Geometry: final body of the model. Coordinates: model frame, mm. Face numbers are marked on the shaded views. A direction names the side the tool comes from. Round coordinates to 2 decimals unless told otherwise and drop trailing zeros. Order: outer loops, then holes, each group sorted by start corner. A loop starts at its lowest first (then second) coordinate and runs counter-clockwise, first axis right, second up. Notation, with made-up numbers: (73.5, -16) -> (128.5, -16) arc R27 cw to (128.5, 8) -> close; hole circle Ø10 at (-34, -5). An arc over 180 degrees is marked (long way). Put each result on its own line as item: value.
```python
from build123d import *

# Parameters (mm, degrees)
SKETCH1_W           = 4
SKETCH1_H           = 76
SKETCH1_H_2         = 4
SKETCH1_W_2         = 76
BOSS_EXTRUDE1_DEPTH = 150


with BuildPart() as part:
    # Sketch1 → Boss-Extrude1 (new body)
    with BuildSketch(Plane.XY):
        with Locations((0, 2)):
            Rectangle(SKETCH1_W, SKETCH1_H)
        with Locations((0, -38)):
            Rectangle(SKETCH1_W, SKETCH1_H_2)
        with Locations((40, -38)):
            Rectangle(SKETCH1_W_2, SKETCH1_H_2)
    extrude(amount=BOSS_EXTRUDE1_DEPTH)


solid = part.part
```
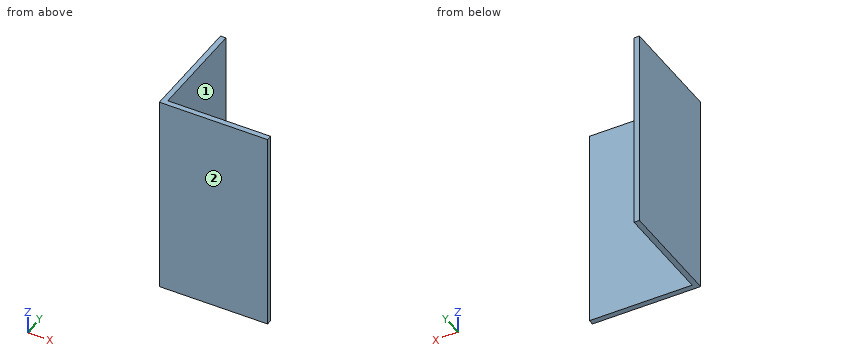
1. Contact query for flat-ended pins moving along their axis: P1, Ø12, axis at x = 52, y = -28, coming from the +Z side; P2, Ø23, axis at y = -4.5, z = 65.5, coming from the +X side; P3, Ø1.5, axis at x = 64, z = 52.5, coming from the +Y side. Output: stop coordinate, or through.
Ans:
P1: through
P2: x = 2
P3: y = -36
2. Material intervals for probe 1 along Y at (x, z) = (62, 119); probe 2 along X at (y, z) = (-29, 136.5), sorted ascending.
Ans:
probe 1: -40 to -36
probe 2: -2 to 2
3. Set-up query: the marked faces 1 and 2. Return all of +Z, -Z, +X, -X, +Y, -Y with unobstructed straight access to the full face (end or side cutting, diameter ignored); none if empty.
Ans:
face 1: +Z, -Z, +X, +Y
face 2: +Z, -Z, +X, -X, -Y
4. Cut plane B-B on y = -20. Return loops of the section in (x, z).
Ans:
outline: (-2, 0) -> (2, 0) -> (2, 150) -> (-2, 150) -> close
5. Cut plane C-C on x = 42. Return loops of the section in (y, z), and give its area (3 significant figures).
Ans:
outline: (-40, 0) -> (-36, 0) -> (-36, 150) -> (-40, 150) -> close
area: 600 mm²
6. Cut plane A-A on z = 102.5. Return loops of the section in (x, y), and give its area (3 significant figures).
Ans:
outline: (-2, -40) -> (78, -40) -> (78, -36) -> (2, -36) -> (2, 40) -> (-2, 40) -> close
area: 624 mm²
